Read the model definition and answer for the solid it produces. Units are mm, in the model's axes. A direction names the side the tool comes from. Round coordinates to 2 decimals unless told otherwise and drop trailing zeros. Order: outer loops, then holes, each group sorted by start corner. A loop starts at its lowest first (then second) coordinate and runs counter-clockwise, first axis right, second up.
from build123d import *

# Parameters (mm, degrees)
BOSS_EXTRUDE1_DEPTH = 7
SKETCH2_W           = 12
SKETCH2_H           = 2.6
CUT_EXTRUDE1_DEPTH  = 7


with BuildPart() as part:
    # Sketch1 → Boss-Extrude1 (new body)
    with BuildSketch(Plane(origin=(0, 0, 0), x_dir=(1, 0, 0), z_dir=(0, 1, 0))):
        Polygon((0, 0), (12, 0), (12, -4.1), (0, -4.1), (0, -8.1), (15, -8.1), (15, 3.9), (1.592592593, 3.9), (0, 3.9), (0, 20), (-4, 20), (-4, 0), align=None)
    extrude(amount=BOSS_EXTRUDE1_DEPTH)

    # Sketch2 → Cut-Extrude1 (cut)
    with BuildSketch(Plane.XY):
        with Locations((6, 1.3)):
            Rectangle(SKETCH2_W, SKETCH2_H)
    extrude(amount=-CUT_EXTRUDE1_DEPTH, mode=Mode.SUBTRACT)


solid = part.part
Q1. A cutting plane is placed at C-C, the plane z = -3.5. Give the vertices of the cut face in (x, y), plus the area to 3 significant figures.
Outcome:
outline: (-4, 0) - (0, 0) - (0, 2.6) - (12, 2.6) - (12, 0) - (15, 0) - (15, 7) - (-4, 7) - close
area: 102 mm2
Q2. Flat-ended cylindrical pins translate along their axes: pin 1 (2 mm diameter, centred on x = 3.5, z = -2, fed in from -Y); pin 2 (3.5 mm diameter, centred on y = 2, z = -7, fed in from +X); pin 3 (2 mm diameter, centred on x = 9.5, y = 5, fed in from -Z). Find the tip coordinate at first contact, or state that the pin passes through.
Outcome:
pin 1: stops at y = 2.6
pin 2: stops at x = 0
pin 3: stops at z = -3.9
Q3. For faces 1 (the face through (0, 3, 6)), 2 (the face through (12, 3, 1)), 3 (the face through (6, 3, 4.1)), determine the directions among +Z, -Z, +X, -X, +Y, -Y from which every point of the face is accessible in a straight line to the end or side of a thin tool.
Outcome:
face 1: +Z, -X, +Y, -Y
face 2: -Y
face 3: -X, +Y, -Y
Q4. For a pull along X with two mould halves and no side action, classify faces 4 (the face through (6, 2.6, -2)), 5 (the face through (15, 3, 2)), 6 (the face through (4, 7, -3)) as released by +X, released by -X, zero draft, split by the parting line, or undercut.
Outcome:
face 4: undercut
face 5: released by +X
face 6: zero draft
Q5. A cutting plane is placed at B-B, the plane x = 11. Give the vertices of the cut face in (y, z), plus the area to 3 significant figures.
Outcome:
outline: (0, 4.1) - (7, 4.1) - (7, 8.1) - (0, 8.1) - close; (2.6, -3.9) - (7, -3.9) - (7, 0) - (2.6, 0) - close
area: 45.2 mm2
Q6. A cutting plane is placed at D-D, the plane y = 6.25. Give the vertices of the cut face in (x, z).
Outcome:
outline: (-4, -20) - (0, -20) - (0, -3.9) - (15, -3.9) - (15, 8.1) - (0, 8.1) - (0, 4.1) - (12, 4.1) - (12, 0) - (-4, 0) - close
Q7. Straight lines are drawn through the part: probe 1 along Z at (x, y) = (0.25, 3.25); probe 2 along X at (y, z) = (6.75, -7.75); probe 3 along X at (y, z) = (1.75, -3.5). For each, find the intervals that lie inside material, in ascending order.
Outcome:
probe 1: z = -3.9 to 0, 4.1 to 8.1
probe 2: x = -4 to 0
probe 3: x = -4 to 0, 12 to 15
Q8. A cutting plane is placed at A-A, the plane y = 2.25. Give the vertices of the cut face in (x, z).
Outcome:
outline: (-4, -20) - (0, -20) - (0, 0) - (-4, 0) - close; (0, 4.1) - (12, 4.1) - (12, -3.9) - (15, -3.9) - (15, 8.1) - (0, 8.1) - close
